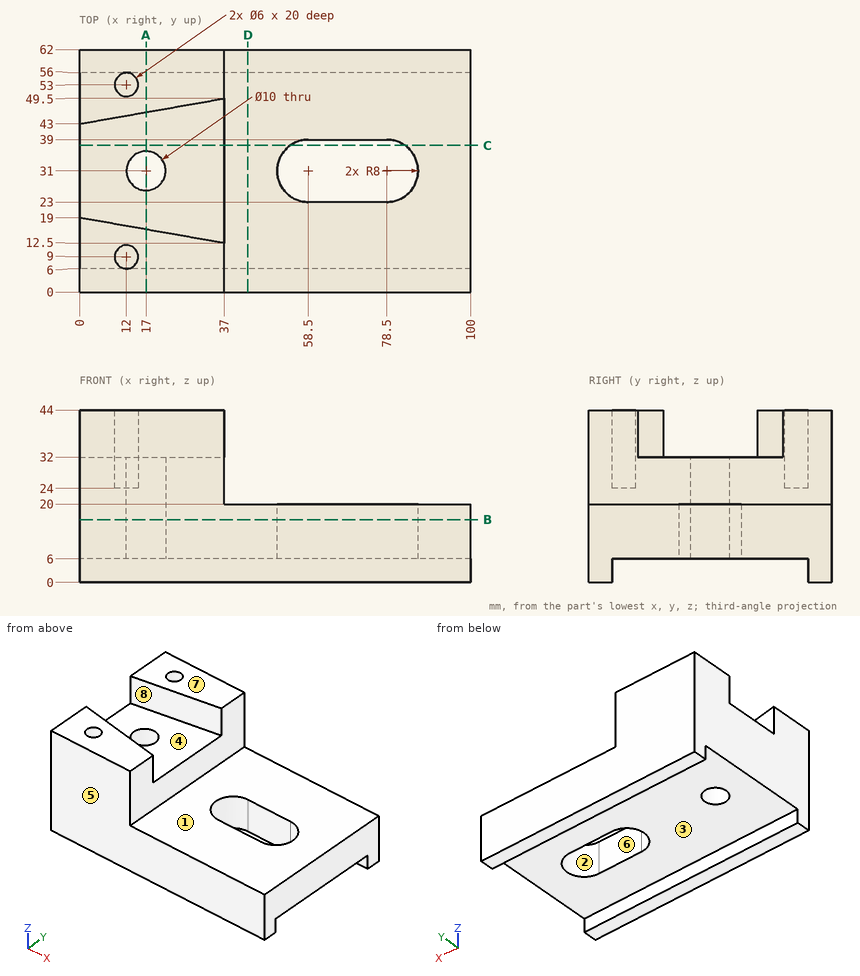
Here's the drawing with two shaded views (mm, measured from the low corner). I have some questions. A direction names the side the tool comes from. Give positions to 0.01 mm unless a question says otherwise; leave off trailing zeros. Order: outer loops, then holes, each group sorted by start corner. A loop starts at its lowest first (then second) coordinate and runs counter-clockwise, first axis right, second up. Notation, with made-up numbers: (56, 32.5) - (80, 32.5) arc R14 cw to (80, 59.5) - close; hole circle Ø11 at (28.25, 6.5). An arc over 180 degrees is marked (long way). Write each question's results on one line, items separated by ' | '.
1) Please list where these lines run through material, in increasing order: line 1 along Z through (x, y) = (24.5, 54); line 2 along Z through (x, y) = (40, 57.5); line 3 along Y through (x, z) = (17, 11.5). Write a range as [from, to].
Final values:
line 1: z = [6, 44] | line 2: z = [0, 20] | line 3: y = [0, 26], [36, 62]
2) On a 3-axis mill with a long thin cutter (end or side, diameter ignored), from which of +Z, -Z, +X, -X, +Y, -Y can I reach the whole of each face in a straight line? I mean the marked faces 1, 2, 3, 4 and 5. Say none if no direction works.
Final values:
face 1: +Z, +X, +Y, -Y | face 2: +Z, -Z | face 3: -Z, +X, -X | face 4: +Z, +X | face 5: +Z, -Z, +X, -X, -Y
3) Suppose I cut it at C-C, the plane y = 37.5. Write out the boundary of the cut face in (x, z), then the cut area to 3 significant figures.
Final values:
outline: (0, 6) - (53.84, 6) - (53.84, 20) - (37, 20) - (37, 32) - (0, 32) - close; (83.16, 6) - (100, 6) - (100, 20) - (83.16, 20) - close | area: 1,430 mm^2
4) Suppose I cut it at B-B, the plane z = 16. Write out the boundary of the cut face in (x, y), then the cut area to 3 significant figures.
Final values:
outline: (0, 0) - (100, 0) - (100, 62) - (0, 62) - close; hole circle Ø10 at (17, 31); hole (58.5, 23) - (78.5, 23) arc R8 ccw to (78.5, 39) - (58.5, 39) arc R8 ccw to start | area: 5,600 mm^2
5) If we mould it in two halves opening along X, with no side actions, what happens to the marked faces 6, 7 and 8? For each: pulls with the +X half, pulls with the -X half, needs draft (parallel to the pull), parting line crosses it, or undercut.
Final values:
face 6: undercut | face 7: needs draft | face 8: pulls with the +X half
6) Suppose I cut it at A-A, the plane x = 17. Write out the boundary of the cut face in (y, z).
Final values:
outline: (0, 0) - (6, 0) - (6, 6) - (26, 6) - (26, 32) - (16.01, 32) - (16.01, 44) - (0, 44) - close; (36, 6) - (56, 6) - (56, 0) - (62, 0) - (62, 44) - (45.99, 44) - (45.99, 32) - (36, 32) - close
7) Suppose I cut it at D-D, the plane x = 43. Write out the boundary of the cut face in (y, z).
Final values:
outline: (0, 0) - (6, 0) - (6, 6) - (56, 6) - (56, 0) - (62, 0) - (62, 20) - (0, 20) - close
8) I'm going to push flat-ended pins straight in: pin 1 Ø1.8 at (x, y) = (13, 10) entering from +Z; pin 2 Ø1.5 at (y, z) = (36.5, 27) entering from +X; pin 3 Ø15 at (x, y) = (71, 42.5) entering from -Z. Where does each tip first touch, or does it pass through?
Final values:
pin 1: stops at z = 24 | pin 2: stops at x = 37 | pin 3: stops at z = 6
